```python
from build123d import *

# Parameters (mm, degrees)
SKETCH1_W           = 54
SKETCH1_H           = 54
BOSS_EXTRUDE1_DEPTH = 26
SKETCH2_R           = 1.70360319
SKETCH2_R_2         = 10
CUT_EXTRUDE1_DEPTH  = 47.19523785
SKETCH3_W           = 54
SKETCH3_H           = 26
BOSS_EXTRUDE2_DEPTH = 20
SKETCH4_W           = 20
SKETCH4_H           = 11
CUT_EXTRUDE2_DEPTH  = 20


with BuildPart() as part:
    # Sketch1 → Boss-Extrude1 (new body)
    with BuildSketch(Plane(origin=(0, 0, 0), x_dir=(1, 0, 0), z_dir=(0, 1, 0))):
        Rectangle(SKETCH1_W, SKETCH1_H)
    extrude(amount=BOSS_EXTRUDE1_DEPTH)

    # Sketch2 → Cut-Extrude1 (cut, through all)
    with BuildSketch(Plane(origin=(0, 26, 0), x_dir=(1, 0, 0), z_dir=(0, 1, 0))):
        with Locations(Location((-6, 22, 0), (0, 0, 270))):
            Circle(SKETCH2_R)
        with Locations(Location((-6, 14, 0), (0, 0, 270))):
            Circle(SKETCH2_R)
        with Locations(Location((19, -5.996588382, 0), (0, 0, 270))):
            Circle(SKETCH2_R)
        with Locations(Location((11, -5.996588382, 0), (0, 0, 270))):
            Circle(SKETCH2_R)
        with Locations(Location((11.896457598, 14, 0), (0, 0, 270))):
            Circle(SKETCH2_R_2)
        with Locations(Location((-6, -5.996588382, 0), (0, 0, 270))):
            Circle(SKETCH2_R_2)
    extrude(amount=-CUT_EXTRUDE1_DEPTH, mode=Mode.SUBTRACT)

    # Sketch3 → Boss-Extrude2 (add)
    with BuildSketch(Plane(origin=(0, 0, -27), x_dir=(-1, 0, 0), z_dir=(0, 0, -1))):
        with Locations((0, 13)):
            Rectangle(SKETCH3_W, SKETCH3_H)
    extrude(amount=BOSS_EXTRUDE2_DEPTH)

    # Sketch4 → Cut-Extrude2 (cut)
    with BuildSketch(Plane(origin=(0, 0, -47), x_dir=(-1, 0, 0), z_dir=(0, 0, -1))):
        with Locations((6, 11.5)):
            Rectangle(SKETCH4_W, SKETCH4_H)
    extrude(amount=-CUT_EXTRUDE2_DEPTH, mode=Mode.SUBTRACT)


solid = part.part
```
Model file for the job. Use its own axes, mm. A direction names the side the tool comes from. Round coordinates to 2 decimals unless told otherwise and drop trailing zeros. Write each loop counter-clockwise with the first axis right and the second up, starting at its lowest first coordinate (ties: lowest second). Pieces come first, ordered by that corner, then holes. Notation, with made-up numbers: (-34, -19.75) -> (-24, -19.75) arc R36 ccw to (-24, 19.25) -> close; hole circle Ø3 at (50, -17.75). An arc over 180 degrees is marked (long way). Answer as CSV lines item,"result".
1. Tool access for faces 4 (the face through (-6, 12, -27)), 5 (the face through (-4.849, 13.182, -15.256)): list every direction of +Z, -Z, +X, -X, +Y, -Y with a clear straight run to the whole face (end or side of a thin tool).
Resolved:
face 4,"-Z"
face 5,"+Y, -Y"
2. Slice it at A-A, the plane x = -6. List the corners of the cut face in (y, z), plus the area to 3 significant figures.
Resolved:
outline,"(0, -47) -> (6, -47) -> (6, -27) -> (17, -27) -> (17, -47) -> (26, -47) -> (26, -23.7) -> (0, -23.7) -> close; (0, -20.3) -> (26, -20.3) -> (26, -15.7) -> (0, -15.7) -> close; (0, -12.3) -> (26, -12.3) -> (26, -4) -> (0, -4) -> close; (0, 16) -> (26, 16) -> (26, 27) -> (0, 27) -> close"
area,"1,010 mm²"
3. Slice it at C-C, the plane z = -40.5. List the corners of the cut face in (x, y).
Resolved:
outline,"(-27, 0) -> (27, 0) -> (27, 26) -> (-27, 26) -> close; hole (-16, 6) -> (4, 6) -> (4, 17) -> (-16, 17) -> close"
4. Slice it at D-D, the plane x = 16. List the corners of the cut face in (y, z), plus the area to 3 significant figures.
Resolved:
outline,"(0, -47) -> (26, -47) -> (26, -23.12) -> (0, -23.12) -> close; (0, -4.88) -> (26, -4.88) -> (26, 27) -> (0, 27) -> close"
area,"1,450 mm²"
5. Mould opens along X. For faces 1 (the face through (-6, 17, -37)), 2 (the face through (-27, 13, -9)), 3 (the face through (0, 0, -9)) say: +X half, -X half, draft (parallel to the pull), parting line (faces both ways), or undercut.
Resolved:
face 1,"undercut"
face 2,"-X half"
face 3,"draft"
6. Slice it at B-B, the plane z = -14. List the corners of the cut face in (x, y).
Resolved:
outline,"(-27, 0) -> (-7.7, 0) -> (-7.7, 26) -> (-27, 26) -> close; (-4.3, 0) -> (1.9, 0) -> (1.9, 26) -> (-4.3, 26) -> close; (21.9, 0) -> (27, 0) -> (27, 26) -> (21.9, 26) -> close"
7. Drill centre lines: line 1 (Y direction, x = -1, z = -32); line 2 (X direction, y = 11, z = -29); line 3 (Z direction, x = -7.5, y = 15.25). Where is each one in solid material? Low to high.
Resolved:
line 1,"0 to 6, 17 to 26"
line 2,"-27 to -16, 4 to 27"
line 3,"-27 to -22.81, -21.19 to -14.81, -13.19 to -3.89, 15.88 to 27"
